For this review, use the dimensioned drawing (mm, ordinates from the lowest corner) and the shaded views. A direction names the side the tool comes from. Round coordinates to 2 decimals unless told otherwise and drop trailing zeros. Loops run counter-clockwise (first coordinate to the right, second up) from the corner with the lowest first, then second, coordinate; pieces in that order, holes last. Notation, with made-up numbers: M 22.5,23.25 L 36.5,23.25 A23 ccw 36.5,45.25 Z; hole C -29,25.25 d5. An arc over 180 degrees is marked long. One line per item, written item: value. Start each with the question number.
Item 1: We need section C-C (x = 74). Write out the cut boundary in (y, z), then the cut area to 3 significant figures.
Item 2: For the marked faces 1, 2 and 3, list the 3-axis set-ups (+Z, -Z, +X, -X, +Y, -Y) from which the entire face can be reached by the end or side of a thin tool; tool diameter is ignored.
Item 3: Clearance check with flat-ended pins moving along their axes: pin 1 (8 mm diameter, centred on x = 37, y = 233, fed in from +Z); pin 2 (10 mm diameter, centred on y = 114, z = 96, fed in from -X); pin 3 (24 mm diameter, centred on x = 59.5, y = 348, fed in from -Z). State where each tip first meets the part, or that it passes through.
Item 4: We need section B-B (z = 25.5). Write out the cut boundary in (x, y).
Item 5: We need section D-D (y = 45.5). Write out the cut boundary in (x, z).
Item 6: Mouldability with a two-part tool opening along Y and no side actions: class the marked faces 4, 5 and 6 as released by +Y, released by -Y, zero draft, split by the parting line, or undercut.
Item 7: For line 1 along Y through (x, z) = (24.5, 31.5); line 2 along X through (y, z) = (429.5, 121); line 3 along Z through (x, y) = (36, 32), list the stretches that pass through material, from the lowest coordinate up.
Item 8: We need section A-A (z = 138.5). Write out the cut boundary in (x, y).
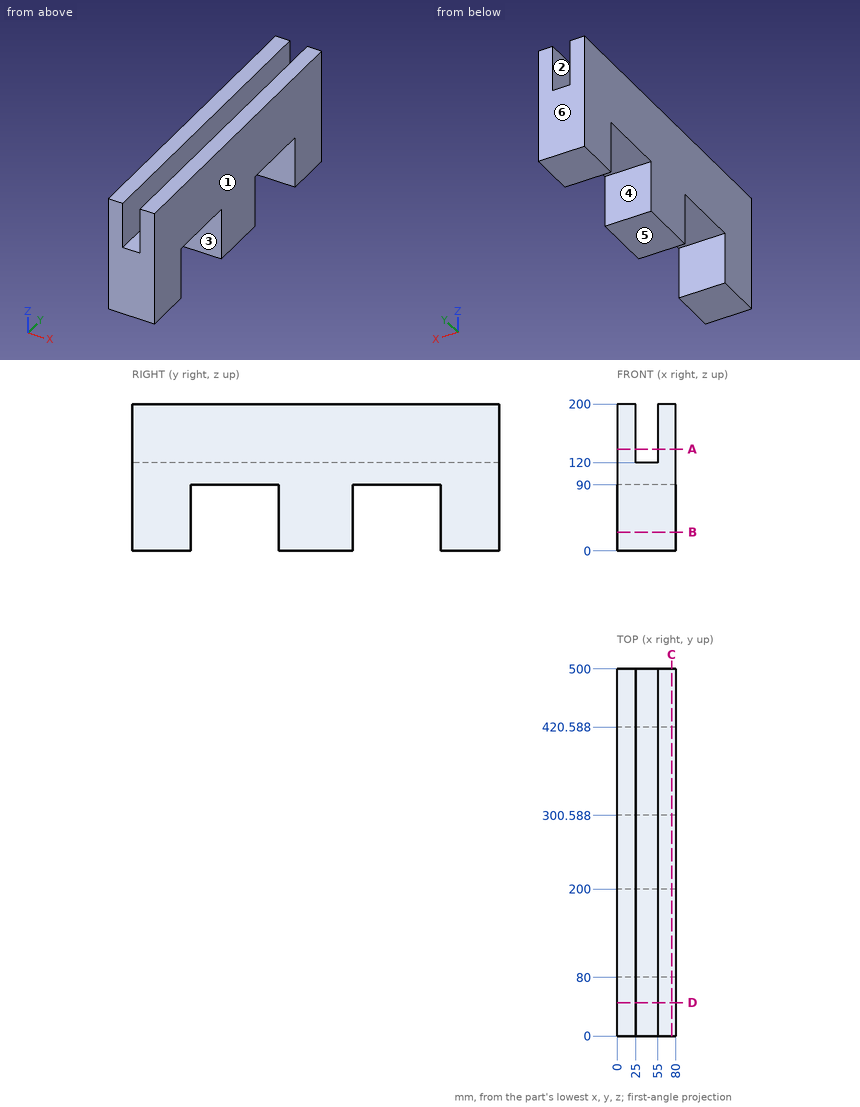
A:
1. outline: M 0,0 L 80,0 L 80,90 L 200,90 L 200,0 L 300.59,0 L 300.59,90 L 420.59,90 L 420.59,0 L 500,0 L 500,200 L 0,200 Z
1. area: 78,400 mm2
2. face 1: +Z, -Z, +X, +Y, -Y
2. face 2: +Z, +Y, -Y
2. face 3: -Z, +X, -X
3. pin 1: z = 120
3. pin 2: x = 0
3. pin 3: z = 90
4. outline: M 0,0 L 80,0 L 80,80 L 0,80 Z; M 0,200 L 80,200 L 80,300.59 L 0,300.59 Z; M 0,420.59 L 80,420.59 L 80,500 L 0,500 Z
5. outline: M 0,0 L 80,0 L 80,200 L 55,200 L 55,120 L 25,120 L 25,200 L 0,200 Z
6. face 4: undercut
6. face 5: zero draft
6. face 6: released by +Y
7. line 1: 0 to 80, 200 to 300.59, 420.59 to 500
7. line 2: 0 to 25, 55 to 80
7. line 3: 0 to 120
8. outline: M 0,0 L 25,0 L 25,500 L 0,500 Z; M 55,0 L 80,0 L 80,500 L 55,500 Z
